from build123d import *

# Parameters (mm, degrees)
F1_DEPTH      = 1920
F3_DEPTH      = 831.201
F3_DEPTH_BACK = 472.271
F4_T          = -3


with BuildPart() as f1:
    # F0 (on Front) → F1 (new body)
    with BuildSketch(Plane.XZ):
        Polygon((-472.27, 737.5), (0, 0), (560, 0), (831.2, 346.48), align=None)
    extrude(amount=-F1_DEPTH)

    # F2 (on Right) → F3 (cut, two sides)
    with BuildSketch(Plane.YZ) as f3_sk:
        Polygon((0, 0), (1920, 0), (1920, 300), align=None)
    extrude(amount=F3_DEPTH, mode=Mode.SUBTRACT)
    extrude(f3_sk.sketch, amount=-F3_DEPTH_BACK, mode=Mode.SUBTRACT)

    # F4
    f4_openings = [f1.faces().sort_by_distance(p)[0] for p in [
        (179.465, 960, 541.99),
    ]]
    offset(amount=F4_T, openings=f4_openings)


solid = f1.part
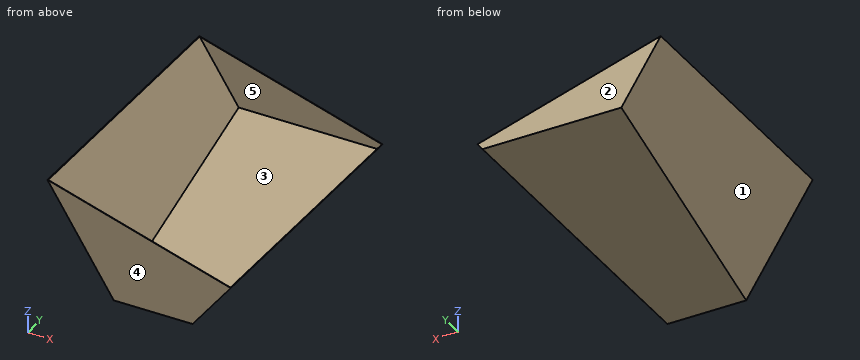
Can you work these out from the model? Positions are in its coordinate system, mm. Face numbers are marked on the shaded views. A direction names the side the tool comes from. Round coordinates to 2 decimals unless told otherwise and drop trailing zeros. Write each loop counter-clockwise with the first axis right and the second up, starting at its lowest first coordinate (ties: lowest second). Pieces come first, ordered by that corner, then holes. Notation, with made-up numbers: (-14, 18) - (20, 18) arc R25 ccw to (20, 55) - close; hole circle Ø6 at (85, 47). An arc over 180 degrees is marked (long way). Write each question's results on one line, items separated by ' | '. Start each with the question number.
1) For pin 1 Ø12 at (y, z) = (315, 136) entering from +X; pin 2 Ø6 at (y, z) = (1045, 248) entering from +X (3 decimals); pin 3 Ø3 at (y, z) = (704.5, 184) entering from +X, each with a flat end and sliding along its axis, tell me the tip position at first contact or that it passes through.
2) Suppose I cut it at C-C (x = -250). List the corners of the cut face in (y, z) for me, and give its area (3 significant figures).
3) Suppose I cut it at B-B (y = 1484.5). List the corners of the cut face in (x, z) for me, and give its area (3 significant figures).
4) Suppose I cut it at A-A (z = 232.5). List the corners of the cut face in (x, y) for me.
5) We'd pull the mould along X, two halves only. Please class the marked faces 1, 2 and 3: released by +X, released by -X, zero draft, split by the parting line, or undercut.
6) Please list where these lines run through material, in increasing order: line 1 (Y direction, x = 83.5, z = 448); line 2 (X direction, y = 722, z = 257.5); line 3 (X direction, y = 765.5, z = 214).
7) Which directions (+Z, -Z, +X, -X, +Y, -Y) give clear straight access to the entire face, cutting with the end or side of a thin tool? Please do the marked faces 4 and 5.
8) Suppose I cut it at D-D (z = 51). List the corners of the cut face in (x, y) for me.
Here are the results:
1) pin 1: stops at x = 671.15 | pin 2: stops at x = 756.465 | pin 3: stops at x = 705.2
2) outline: (0, 390.4) - (1920, 390.4) - (1920, 670.82) - (1917, 670.82) - (1917, 395.96) - (3, 395.96) - (3, 670.82) - (0, 670.82) - close | area: 12,300 mm2
3) outline: (-472.27, 737.5) - (-148.53, 231.95) - (741.56, 231.95) - (831.2, 346.48) - (828.11, 347.41) - (740.12, 234.99) - (-146.92, 234.99) - (-467.86, 736.18) - close | area: 4,920 mm2
4) outline: (-148.89, 0) - (741.98, 0) - (741.98, 1488) - (-148.89, 1488) - close; hole (-145.32, 3) - (738.17, 3) - (738.17, 1468.57) - (-145.32, 1468.57) - close
5) face 1: released by -X | face 2: zero draft | face 3: undercut
6) line 1: y = 0 to 3, 1917 to 1920 | line 2: x = -164.89 to -161.33, 757.74 to 761.55 | line 3: x = -137.04 to -133.48, 723.69 to 727.5
7) face 4: +Z, -Z, +X, -X, -Y | face 5: +Z
8) outline: (-32.66, 0) - (599.92, 0) - (599.92, 326.4) - (-32.66, 326.4) - close; hole (-29.1, 3) - (596.11, 3) - (596.11, 306.97) - (-29.1, 306.97) - close
